The listing builds one solid part. Answer for the finished solid, in the listing's coordinates (mm). A direction names the side the tool comes from. Coordinates: 2 decimals unless noted, no trailing zeros. Order: outer loops, then holes, each group sorted by start corner. A loop starts at its lowest first (then second) coordinate and runs counter-clockwise, first axis right, second up.
from build123d import *

# Parameters (mm, degrees)
EXTRUDE_1_DEPTH     = 10
SKETCH_3_R          = 10.75
CUT_EXTRUDE_1_DEPTH = 55.591666031
SKETCH_4_R          = 1.5
CUT_EXTRUDE_2_DEPTH = 55.591666031
FILLET_1_R          = 10
FILLET_3_R          = 3
SKETCH_7_W          = 22
SKETCH_7_H          = 13
CUT_EXTRUDE_5_DEPTH = 55.591666031
FILLET_4_R          = 3
SKETCH_8_W          = 9
SKETCH_8_H          = 5
EXTRUDE_2_DEPTH     = 10
FILLET_5_R          = 1
SKETCH_9_R          = 1.5
CUT_EXTRUDE_6_DEPTH = 5


with BuildPart() as part:
    # 草图2 → 凸台-拉伸1 (new body)
    with BuildSketch(Plane.XY):
        Polygon((30, 0), (-30, 0), (-30, 15), (-16, 15), (-16, 44.5), (16, 44.5), (16, 15), (30, 15), align=None)
    extrude(amount=EXTRUDE_1_DEPTH)

    # 草图3 → 切除-拉伸1 (cut, through all)
    with BuildSketch(Plane.XY.offset(10)):
        with Locations((0, 44.5)):
            Circle(SKETCH_3_R)
    extrude(amount=-CUT_EXTRUDE_1_DEPTH, mode=Mode.SUBTRACT)

    # 草图4 → 切除-拉伸2 (cut, through all)
    with BuildSketch(Plane.XY.offset(10)):
        with Locations((-20, 7.5)):
            Circle(SKETCH_4_R)
        with Locations((0, 7.5)):
            Circle(SKETCH_4_R)
        with Locations((20, 7.5)):
            Circle(SKETCH_4_R)
    extrude(amount=-CUT_EXTRUDE_2_DEPTH, mode=Mode.SUBTRACT)

    # 圆角1
    fillet_1_edges = [part.edges().sort_by_distance(p)[0] for p in [
        (-16, 15, 5),
        (16, 15, 5),
    ]]
    fillet(fillet_1_edges, radius=FILLET_1_R)

    # 圆角3
    fillet_3_edges = [part.edges().sort_by_distance(p)[0] for p in [
        (-30, 15, 5),
        (30, 15, 5),
    ]]
    fillet(fillet_3_edges, radius=FILLET_3_R)

    # 草图7 → 切除-拉伸5 (cut, through all)
    with BuildSketch(Plane.XY.offset(10)):
        with Locations((0, 21.5)):
            Rectangle(SKETCH_7_W, SKETCH_7_H)
    extrude(amount=-CUT_EXTRUDE_5_DEPTH, mode=Mode.SUBTRACT)

    # 圆角4
    fillet_4_edges = [part.edges().sort_by_distance(p)[0] for p in [
        (11, 28, 5),
        (11, 15, 5),
        (-11, 15, 5),
        (-11, 28, 5),
    ]]
    fillet(fillet_4_edges, radius=FILLET_4_R)

    # 草图8 → 凸台-拉伸2 (add)
    with BuildSketch(Plane.XY.offset(10)):
        with Locations((20.5, 42)):
            Rectangle(SKETCH_8_W, SKETCH_8_H)
        with Locations((-20.5, 42)):
            Rectangle(SKETCH_8_W, SKETCH_8_H)
    extrude(amount=-EXTRUDE_2_DEPTH)

    # 圆角5
    fillet_5_edges = [part.edges().sort_by_distance(p)[0] for p in [
        (-16, 39.5, 5),
        (16, 39.5, 5),
    ]]
    fillet(fillet_5_edges, radius=FILLET_5_R)

    # 草图9 → 切除-拉伸6 (cut)
    with BuildSketch(Plane(origin=(0, 44.5, 0), x_dir=(1, 0, 0), z_dir=(0, 1, 0))):
        with Locations(Location((-21, -5, 0), (0, 0, 270))):
            Circle(SKETCH_9_R)
        with Locations(Location((21, -5, 0), (0, 0, 90))):
            Circle(SKETCH_9_R)
    extrude(amount=-CUT_EXTRUDE_6_DEPTH, mode=Mode.SUBTRACT)


solid = part.part
(1) Find section C-C on z = 8. Count the separate pieces of the cut face and the enclosed holes in it, then the cut area to 3 significant figures.
(2) The mould has two halves that part along X. Classify faces 5 (the cylindrical face through (-29.14, 14.1, 5.07)), 6 (the cylindrical face through (10.14, 15.9, 4.93)), 7 (the flat face through (18, 44.5, 5)): pulls with the +X half, pulls with the -X half, needs draft (parallel to the pull), parting line crosses it, or undercut.
(3) A tool of negligible diameter and unlimited length cuts with its end or side. For faces 1 (the flat face through (11, 21, 5)), 2 (the flat face through (-16, 32, 5)), 3 (the cylindrical face through (-19.735, 42.035, 5.806)), 4 (the flat face through (16, 32, 5)), from which of +Z, -Z, +X, -X, +Y, -Y can it reach the whole face along a straight path? Write none if from no direction.
(4) Given pin 1 Ø2 at (y, z) = (21, 4.5) entering from -X; pin 2 Ø1.5 at (y, z) = (41, 7) entering from -X; pin 3 Ø0.5 at (x, z) = (26.5, 4) entering from +Y; pin 4 Ø2.5 at (x, y) = (-20, 7.5) entering from -Z, each flat-ended and moving along its own axis, determine where each tip first touches the part or whether it passes through.
(5) Find section A-A on y = 19. Determine the outline of the cut face in (x, z), then the cut area to 3 significant figures.
(6) Find the intervals of material crossed by probe 1 along X at (y, z) = (41.5, 6.25); probe 2 along Z at (x, y) = (21, 42); probe 3 along X at (y, z) = (30.5, 6), in increasing order.
(7) Find section B-B on x = 6. Determine the outline of the cut face in (y, z).
Resolved:
1. separate pieces: 1
1. enclosed holes: 4
1. area: 1,490 mm2
2. face 5: pulls with the -X half
2. face 6: undercut
2. face 7: needs draft
3. face 1: +Z, -Z
3. face 2: +Z, -Z, -X
3. face 3: +Y
3. face 4: +Z, -Z, +X
4. pin 1: stops at x = -17.34
4. pin 2: stops at x = -25
4. pin 3: stops at y = 15
4. pin 4: passes through
5. outline: (-18, 0) - (-11, 0) - (-11, 10) - (-18, 10) - close; (11, 0) - (18, 0) - (18, 10) - (11, 10) - close
5. area: 140 mm2
6. probe 1: x = -25 to -21.83, -20.17 to -10.32, 10.32 to 20.17, 21.83 to 25
6. probe 2: z = 0 to 3.5, 6.5 to 10
6. probe 3: x = -16 to 16
7. outline: (0, 0) - (15, 0) - (15, 10) - (0, 10) - close; (28, 0) - (35.58, 0) - (35.58, 10) - (28, 10) - close
